Check sheet for the modelled part. Datum: model origin and axes. Units: mm. Coordinates: 2 decimals unless noted, no trailing zeros. Order: outer loops, then holes, each group sorted by start corner. A loop starts at its lowest first (then second) coordinate and runs counter-clockwise, first axis right, second up.
1. Draft check along X on faces 1 (the flat face through (-38, 1, 0)), 2 (the cylindrical face through (-70.93, 1.17, -16.54)), 3 (the cylindrical face through (-70.382, 1.174, -106.493)), 4 (the flat face through (-76.2, 1, -60)). Enter one of: released by +X, released by -X, zero draft, split by the parting line, or undercut.
2. Thickness scan on line 1 (Z direction, x = -12.7, y = 1.15); line 2 (Z direction, x = -12.5, y = 0.5); line 3 (X direction, y = 0.95, z = -106). Record the ranges inside material, lowest first.
3. Cross-section at A-A (x = -12.7). Enter the section's corners in (y, z).
Autodesk Inventor part; units mm, degrees
ref_plane "YZ Plane" through (0, 0, 0) normal (1, 0, 0) x (0, 1, 0)
ref_plane "XZ Plane" through (0, 0, 0) normal (0, 1, 0) x (-1, 0, 0)
ref_plane "XY Plane" through (0, 0, 0) normal (0, 0, 1) x (1, 0, 0)
sketch "Sketch1" plane through (0, 0, 0) normal (0, 1, 0) x (-1, 0, 0)
  line L0 (0, 0) -> (76.2, 0)
  line L1 (76.2, 0) -> (76.2, -121.539)
  line L2 (76.2, -121.539) -> (0, -121.539)
  line L3 (0, -121.539) -> (0, 0)
  dimension "d0" = 76.2
  dimension "d1" = 121.539
extrude "Extrusion1" add sketch "Sketch1" along normal blind 2.3813
sketch "Sketch2" plane through (0, 2.3813, 0) normal (0, 1, 0) x (1, 0, 0)
  line L0 (-6.985, -6.7053) -> (-6.985, 140.88) construction
  line L1 (-69.215, -6.7053) -> (-69.215, 134.4303) construction
  line L2 (-84.4429, 16.3195) -> (15.1684, 16.3195) construction
  line L3 (-82.9542, 105.2195) -> (32.716, 105.2195) construction
  line L4 (-85.3039, 60.7695) -> (24.2122, 60.7695) construction
  line L5 (-38.1, -11.6346) -> (-38.1, 148.7845) construction
  line L6 (-76.2, 121.539) -> (-76.2, 0) construction
  line L7 (-76.2, 0) -> (0, 0) construction
  point P0 (-76.2, 60.7695)
  point P1 (-38.1, 0)
  point P2 (-69.215, 16.3195)
  point P3 (-6.985, 16.3195)
  point P4 (-6.985, 105.2195)
  point P5 (-69.215, 105.2195)
  dimension "d4" = 88.9
  dimension "d5" = 62.23
hole "Hole1" at (-69.215, 2.3813, -16.3195) at (-6.985, 2.3813, -16.3195) at (-6.985, 2.3813, -105.2195) at (-69.215, 2.3813, -105.2195) direction (0, -1, 0) diameter 3.4544 depth 25.4 tip angle 118
sketch "Sketch3" plane through (0, 2.3813, 0) normal (0, 1, 0) x (1, 0, 0)
  line L0 (-12.7, -7.2404) -> (-12.7, 131.1471) construction
  line L1 (0, 0) -> (0, 121.539) construction
  line L2 (-88.3446, 60.7695) -> (40.5312, 60.7695) construction
  point P0 (-12.7, 6.7945)
  point P1 (-12.7, 114.7445)
  point P2 (0, 60.7695)
  dimension "d13" = 12.7
  dimension "d14" = 107.95
hole "Hole2" at (-12.7, 2.3813, -6.7945) at (-12.7, 2.3813, -114.7445) direction (0, -1, 0) diameter 3.81 depth 25.4 tip angle 118
properties part number "redboard_plate"
Data:
1. face 1: zero draft
1. face 2: undercut
1. face 3: undercut
1. face 4: released by -X
2. line 1: z = -121.54 to -116.65, -112.84 to -8.7, -4.89 to 0
2. line 2: z = -121.54 to -116.64, -112.85 to -8.69, -4.9 to 0
2. line 3: x = -76.2 to -70.76, -67.67 to -8.53, -5.44 to 0
3. outline: (0, -121.54) - (2.38, -121.54) - (2.38, -116.65) - (0, -116.65) - close; (0, -112.84) - (2.38, -112.84) - (2.38, -8.7) - (0, -8.7) - close; (0, -4.89) - (2.38, -4.89) - (2.38, 0) - (0, 0) - close
